from build123d import *
from OCP.BRepFilletAPI import BRepFilletAPI_MakeChamfer

# Parameters (mm, degrees)
SKETCH1_R                = 3.1
BOSS_EXTRUDE1_DEPTH      = 12
CHAMFER1_SIZE            = 0.5
CHAMFER1_SIZE2           = 0.714074003
BOSS_EXTRUDE2_DEPTH      = 0.5
BOSS_EXTRUDE2_DEPTH_BACK = 0.5


with BuildPart() as part:
    # Sketch1 → Boss-Extrude1 (new body)
    with BuildSketch(Plane.XY):
        Circle(SKETCH1_R)
    extrude(amount=BOSS_EXTRUDE1_DEPTH)

    # Chamfer1: one chamfer whose edges measure the first distance from different faces: ONE call of the kernel's chamfer builder (chamfer() names one face for all edges)
    chamfer1_edges_1 = [part.edges().sort_by_distance(p)[0] for p in [
        (-3.1, 0, 0),
    ]]
    chamfer1_side_1 = [part.faces().sort_by_distance(p)[0] for p in [
        (0, 0, 0),
    ]]
    chamfer1_edges_2 = [part.edges().sort_by_distance(p)[0] for p in [
        (-3.1, 0, 12),
    ]]
    chamfer1_side_2 = [part.faces().sort_by_distance(p)[0] for p in [
        (-3.1, 0, 6),
    ]]
    chamfer1 = BRepFilletAPI_MakeChamfer(part.part.solid().wrapped)
    for e in chamfer1_edges_1:
        chamfer1.Add(CHAMFER1_SIZE, CHAMFER1_SIZE2, e.wrapped, chamfer1_side_1[0].wrapped)  # the first distance lies on this face
    for e in chamfer1_edges_2:
        chamfer1.Add(CHAMFER1_SIZE, CHAMFER1_SIZE2, e.wrapped, chamfer1_side_2[0].wrapped)  # the first distance lies on this face
    add(Compound.cast(chamfer1.Shape()), mode=Mode.REPLACE)

    # Sketch2 → Boss-Extrude2 (add, two sides: drawn at the far end of the back side and taken through both)
    with BuildSketch(Plane.XY.offset(6).offset(-BOSS_EXTRUDE2_DEPTH_BACK)):
        with BuildLine():
            Line((-6.34428877, -4), (6.34428877, -4))
            ThreePointArc((6.34428877, -4), (0, 7.5), (-6.34428877, -4))
        make_face()
    extrude(amount=BOSS_EXTRUDE2_DEPTH + BOSS_EXTRUDE2_DEPTH_BACK)


solid = part.part
Work out the finished part from the listing and answer in its coordinate system (mm). A direction names the side the tool comes from. Coordinates: 2 decimals unless noted, no trailing zeros. Loops run counter-clockwise (first coordinate to the right, second up) from the corner with the lowest first, then second, coordinate; pieces in that order, holes last. Notation, with made-up numbers: M -37,20 L 17,20 A25 cw 17,44 Z; hole C 50,34 d9. An arc over 180 degrees is marked long. Answer in a Markdown table with one row per item. Add a question column.
1. Flat-ended cylindrical pins translate along their axes: P1, Ø1, axis at y = 1, z = 9, coming from the +X side; P2, Ø3, axis at y = 5.5, z = 5.5, coming from the -X side. Find the tip coordinate at first contact, or state that the pin passes through.
2. A tool of negligible diameter and unlimited length cuts with its end or side. For faces 1 (the flat face through (0, 0, 0)), 2 (the cylindrical face through (1.43, -2.75, 8.96)), 3 (the cylindrical face through (1.43, -2.75, 3.07)), from which of +Z, -Z, +X, -X, +Y, -Y can it reach the whole face along a straight path? Write none if from no direction.
3. Find section C-C, the plane z = 8.5. Write down the section's boundary in (x, y), then the cut area to 3 significant figures.
4. Consider L1, parallel to Z at x = 7, y = 1.5; L2, parallel to X at y = 0, z = 10.5; L3, parallel to X at y = 1.75, z = 2. Determine where each line is inside the solid, lowest interval first.
5. Find section D-D, the plane x = 4.5. Write down the section's boundary in (y, z).
6. Find section A-A, the plane x = 0. Write down the section's boundary in (y, z), then the cut area to 3 significant figures.
7. Find section B-B, the plane y = 0. Write down the section's boundary in (x, z), then the cut area to 3 significant figures.
Reported:
| question | item | result |
|---|---|---|
| 1 | P1 | stops at x = 3.06 |
| 1 | P2 | stops at x = -6.34 |
| 2 | face 1 | -Z, +X, -X, +Y, -Y |
| 2 | face 2 | +Z |
| 2 | face 3 | -Z |
| 3 | outline | C 0,0 d6.2 |
| 3 | area | 30.2 mm^2 |
| 4 | L1 | z = 5.5 to 6.5 |
| 4 | L2 | x = -3.1 to 3.1 |
| 4 | L3 | x = -2.56 to 2.56 |
| 5 | outline | M -4,5.5 L 6,5.5 L 6,6.5 L -4,6.5 Z |
| 6 | outline | M -4,5.5 L -3.1,5.5 L -3.1,0.71 L -2.6,0 L 2.6,0 L 3.1,0.71 L 3.1,5.5 L 7.5,5.5 L 7.5,6.5 L 3.1,6.5 L 3.1,11.5 L 2.39,12 L -2.39,12 L -3.1,11.5 L -3.1,6.5 L -4,6.5 Z |
| 6 | area | 79.0 mm^2 |
| 7 | outline | M -7.5,5.5 L -3.1,5.5 L -3.1,0.71 L -2.6,0 L 2.6,0 L 3.1,0.71 L 3.1,5.5 L 7.5,5.5 L 7.5,6.5 L 3.1,6.5 L 3.1,11.5 L 2.39,12 L -2.39,12 L -3.1,11.5 L -3.1,6.5 L -7.5,6.5 Z |
| 7 | area | 82.5 mm^2 |
